from build123d import *

# Parameters (mm, degrees)
ESQUISSE1_R              = 80
BOSS_EXTRU_1_DEPTH       = 3
ESQUISSE2_R              = 1
ENL_V_MAT_EXTRU_1_DEPTH  = 3
ESQUISSE3_R              = 1.5
ENL_V_MAT_EXTRU_10_DEPTH = 3


with BuildPart() as part:
    # Esquisse1 → Boss.-Extru.1 (new body)
    with BuildSketch(Plane.XY):
        with Locations((-11.197924537, 8.24446622)):
            Circle(ESQUISSE1_R)
    extrude(amount=BOSS_EXTRU_1_DEPTH)

    # Esquisse2 → Enlèv. mat.-Extru.1 (cut)
    # profile 1 of 2: a face of its own
    with BuildSketch(Plane(origin=(0, 0, 0), x_dir=(-1, 0, 0), z_dir=(0, 0, -1))):
        Polygon((-3.802075463, 11.24446622), (-3.802075463, 5.24446622), (1.197924537, 5.24446622), (1.197924537, -2.25553378), (42.197924537, -2.25553378), (42.197924537, 18.74446622), (1.197924537, 18.74446622), (1.197924537, 11.24446622), align=None)
        with Locations((11.197924537, 8.24446622)):
            Circle(ESQUISSE2_R, mode=Mode.SUBTRACT)
    # profile 2 of 2: a face of its own
    with BuildSketch(Plane(origin=(0, 0, 0), x_dir=(-1, 0, 0), z_dir=(0, 0, -1))):
        with Locations((11.197924537, 8.24446622)):
            Circle(ESQUISSE2_R)
    extrude(amount=-ENL_V_MAT_EXTRU_1_DEPTH, mode=Mode.SUBTRACT)

    # Esquisse3 → Enlèv. mat.-Extru.10 (cut)
    with BuildSketch(Plane(origin=(0, 0, 0), x_dir=(-1, 0, 0), z_dir=(0, 0, -1))):
        with BuildLine():
            ThreePointArc((36.197924537, -40.917518651), (28.875594067, -23.239849121), (11.197924537, -15.917518651))
            Line((11.197924537, -15.917518651), (11.197924537, -65.917518651))
            ThreePointArc((11.197924537, -65.917518651), (28.875594067, -58.59518818), (36.197924537, -40.917518651))
        make_face()
        with BuildLine():
            Line((11.197924537, -65.917518651), (11.197924537, -15.917518651))
            ThreePointArc((11.197924537, -15.917518651), (-13.802075463, -40.917518651), (11.197924537, -65.917518651))
        make_face()
        with Locations((-8.802075463, -65.919884489)):
            Circle(ESQUISSE3_R)
        with Locations((31.197924537, -65.917518651)):
            Circle(ESQUISSE3_R)
    extrude(amount=-ENL_V_MAT_EXTRU_10_DEPTH, mode=Mode.SUBTRACT)


solid = part.part
Build history of the part. All positions in model axes, mm. Round coordinates to 2 decimals unless told otherwise and drop trailing zeros. Write each loop counter-clockwise with the first axis right and the second up, starting at its lowest first coordinate (ties: lowest second). Pieces come first, ordered by that corner, then holes. Notation, with made-up numbers: M -31,-9 L -23,-9 A23 cw -23,10 Z; hole C 13.25,-2 d2. An arc over 180 degrees is marked long. Answer as a JSON object with one key per item and string values. Group by question number.
(1) Cut at D-D (x = -52). Give the cut face in (y, z).
(2) Cut at B-B (x = -26). Give the cut face in (y, z).
(3) Drill centre lines: L1, parallel to Y at x = -8.5, z = 0.8; L2, parallel to Y at x = 5, z = 2.45; L3, parallel to Y at x = 4, z = 2.95. Where is each one in solid material? Low to high.
(4) Cut at A-A (z = 2.5). Give the cut face in (x, y).
(5) Flat gauge pins, fed straight in: pin 1 (0.9 mm diameter, centred on x = 0.5, z = 1, fed in from -Y); pin 2 (0.9 mm diameter, centred on x = -30, z = 1.5, fed in from +Y); pin 3 (1.5 mm diameter, centred on x = 2.5, z = 1, fed in from +Y). Where does each tip first touch, or does it go through?
(6) Cut at C-C (y = 69.5). Give the cut face in (x, z), and give its area (3 significant figures).
Responses:
{
 "1": {"outline": "M -60.57,0 L 77.06,0 L 77.06,3 L -60.57,3 Z"},
 "2": {"outline": "M -70.37,0 L -61.06,0 L -61.06,3 L -70.37,3 Z; M -20.77,0 L -2.26,0 L -2.26,3 L -20.77,3 Z; M 18.74,0 L 86.86,0 L 86.86,3 L 18.74,3 Z"},
 "3": {"L1": "y = -71.71 to -65.77, -16.06 to -2.26, 18.74 to 88.2", "L2": "y = -70.1 to -59.96, -21.87 to 86.59", "L3": "y = -70.3 to -60.77, -21.07 to 86.79"},
 "4": {"outline": "C -11.2,8.24 d160; hole M -42.2,-2.26 L -1.2,-2.26 L -1.2,5.24 L 3.8,5.24 L 3.8,11.24 L -1.2,11.24 L -1.2,18.74 L -42.2,18.74 Z; hole C -11.2,-40.92 d50; hole C -31.2,-65.92 d3; hole C 8.8,-65.92 d3"},
 "5": {"pin 1": "stops at y = -70.96", "pin 2": "stops at y = 86.11", "pin 3": "stops at y = 87.19"},
 "6": {"outline": "M -62.65,0 L 40.26,0 L 40.26,3 L -62.65,3 Z", "area": "309 mm2"}
}
